Input: part model. Units: mm. Frame: model coordinates. A direction names the side the tool comes from. Coordinates: 2 decimals unless noted, no trailing zeros. Order: outer loops, then holes, each group sorted by start corner. A loop starts at its lowest first (then second) coordinate and runs counter-clockwise, first axis right, second up. Notation, with made-up numbers: M 34.5,34 L 67.5,34 A22 cw 67.5,71 Z; hole C -38,15.5 d4. An arc over 180 degrees is marked long. One line per item, written item: value.
```python
from build123d import *

# Parameters (mm, degrees)
SKETCH_1_R               = 130
SKETCH_1_R_2             = 30
SKETCH_1_R_3             = 2.1
SKETCH_1_R_4             = 1.6
EXTRUDE_1_DEPTH          = 5
SKETCH_2_R               = 1.4
CUT_EXTRUDE_1_DEPTH      = 1
CUT_EXTRUDE_1_DEPTH_BACK = 6
CUT_EXTRUDE_2_REACH      = 7
SKETCH_8_R               = 1.6
CUT_EXTRUDE_3_DEPTH      = 314.847763109


with BuildPart() as part:
    # 草图1 → 凸台-拉伸1 (new body)
    with BuildSketch(Plane.XY):
        Circle(SKETCH_1_R)
        Circle(SKETCH_1_R_2, mode=Mode.SUBTRACT)
        with Locations((0, 120)):
            Circle(SKETCH_1_R_3, mode=Mode.SUBTRACT)
        with Locations((120, 0)):
            Circle(SKETCH_1_R_3, mode=Mode.SUBTRACT)
        with Locations((0, -120)):
            Circle(SKETCH_1_R_3, mode=Mode.SUBTRACT)
        with Locations((-120, 0)):
            Circle(SKETCH_1_R_3, mode=Mode.SUBTRACT)
        with Locations((0, 40)):
            Circle(SKETCH_1_R_4, mode=Mode.SUBTRACT)
        with Locations((40, 0)):
            Circle(SKETCH_1_R_4, mode=Mode.SUBTRACT)
        with Locations((0, -40)):
            Circle(SKETCH_1_R_4, mode=Mode.SUBTRACT)
        with Locations((-40, 0)):
            Circle(SKETCH_1_R_4, mode=Mode.SUBTRACT)
    extrude(amount=EXTRUDE_1_DEPTH)

    # 草图2 → 切除-拉伸1 (cut, two sides)
    with BuildSketch(Plane.XY.offset(5)) as cut_extrude_1_sk:
        with Locations((0, 95)):
            Circle(SKETCH_2_R)
        with Locations((15, 80)):
            Circle(SKETCH_2_R)
        with Locations((0, 65)):
            Circle(SKETCH_2_R)
        with Locations((-15, 80)):
            Circle(SKETCH_2_R)
        with Locations((95, 0)):
            Circle(SKETCH_2_R)
        with Locations((80, -15)):
            Circle(SKETCH_2_R)
        with Locations((65, 0)):
            Circle(SKETCH_2_R)
        with Locations((80, 15)):
            Circle(SKETCH_2_R)
        with Locations((0, -95)):
            Circle(SKETCH_2_R)
        with Locations((-15, -80)):
            Circle(SKETCH_2_R)
        with Locations((0, -65)):
            Circle(SKETCH_2_R)
        with Locations((15, -80)):
            Circle(SKETCH_2_R)
        with Locations((-95, 0)):
            Circle(SKETCH_2_R)
        with Locations((-80, 15)):
            Circle(SKETCH_2_R)
        with Locations((-65, 0)):
            Circle(SKETCH_2_R)
        with Locations((-80, -15)):
            Circle(SKETCH_2_R)
    extrude(amount=CUT_EXTRUDE_1_DEPTH, mode=Mode.SUBTRACT)
    extrude(cut_extrude_1_sk.sketch, amount=-CUT_EXTRUDE_1_DEPTH_BACK, mode=Mode.SUBTRACT)

    # 草图8 → 切除-拉伸2 (cut, up to next)
    with BuildSketch(Plane(origin=(0, 0, 0), x_dir=(-1, 0, 0), z_dir=(0, 0, -1)), mode=Mode.PRIVATE) as cut_extrude_2_sk1:
        with Locations((-75.840860977, 86.447462694)):
            Circle(SKETCH_8_R)
    cut_extrude_2_tool1 = extrude(cut_extrude_2_sk1.sketch, amount=-CUT_EXTRUDE_2_REACH, mode=Mode.PRIVATE) & part.part
    add(cut_extrude_2_tool1.solids().sort_by_distance((75.840861, 86.447463, 0))[0], mode=Mode.SUBTRACT)
    # 草图8 → 切除-拉伸2 (cut, up to next)
    with BuildSketch(Plane(origin=(0, 0, 0), x_dir=(-1, 0, 0), z_dir=(0, 0, -1)), mode=Mode.PRIVATE) as cut_extrude_2_sk2:
        with Locations((-86.447462694, 75.840860977)):
            Circle(SKETCH_8_R)
    cut_extrude_2_tool2 = extrude(cut_extrude_2_sk2.sketch, amount=-CUT_EXTRUDE_2_REACH, mode=Mode.PRIVATE) & part.part
    add(cut_extrude_2_tool2.solids().sort_by_distance((86.447463, 75.840861, 0))[0], mode=Mode.SUBTRACT)
    # 草图8 → 切除-拉伸2 (cut, up to next)
    with BuildSketch(Plane(origin=(0, 0, 0), x_dir=(-1, 0, 0), z_dir=(0, 0, -1)), mode=Mode.PRIVATE) as cut_extrude_2_sk3:
        with Locations((-65.948574762, 75.171706691)):
            Circle(SKETCH_8_R)
    cut_extrude_2_tool3 = extrude(cut_extrude_2_sk3.sketch, amount=-CUT_EXTRUDE_2_REACH, mode=Mode.PRIVATE) & part.part
    add(cut_extrude_2_tool3.solids().sort_by_distance((65.948575, 75.171707, 0))[0], mode=Mode.SUBTRACT)
    # 草图8 → 切除-拉伸2 (cut, up to next)
    with BuildSketch(Plane(origin=(0, 0, 0), x_dir=(-1, 0, 0), z_dir=(0, 0, -1)), mode=Mode.PRIVATE) as cut_extrude_2_sk4:
        with Locations((-75.171706691, 65.948574762)):
            Circle(SKETCH_8_R)
    cut_extrude_2_tool4 = extrude(cut_extrude_2_sk4.sketch, amount=-CUT_EXTRUDE_2_REACH, mode=Mode.PRIVATE) & part.part
    add(cut_extrude_2_tool4.solids().sort_by_distance((75.171707, 65.948575, 0))[0], mode=Mode.SUBTRACT)
    # 草图8 → 切除-拉伸2 (cut, up to next)
    with BuildSketch(Plane(origin=(0, 0, 0), x_dir=(-1, 0, 0), z_dir=(0, 0, -1)), mode=Mode.PRIVATE) as cut_extrude_2_sk5:
        with Locations((65.948574762, -75.171706691)):
            Circle(SKETCH_8_R)
    cut_extrude_2_tool5 = extrude(cut_extrude_2_sk5.sketch, amount=-CUT_EXTRUDE_2_REACH, mode=Mode.PRIVATE) & part.part
    add(cut_extrude_2_tool5.solids().sort_by_distance((-65.948575, -75.171707, 0))[0], mode=Mode.SUBTRACT)
    # 草图8 → 切除-拉伸2 (cut, up to next)
    with BuildSketch(Plane(origin=(0, 0, 0), x_dir=(-1, 0, 0), z_dir=(0, 0, -1)), mode=Mode.PRIVATE) as cut_extrude_2_sk6:
        with Locations((75.171706691, -65.948574762)):
            Circle(SKETCH_8_R)
    cut_extrude_2_tool6 = extrude(cut_extrude_2_sk6.sketch, amount=-CUT_EXTRUDE_2_REACH, mode=Mode.PRIVATE) & part.part
    add(cut_extrude_2_tool6.solids().sort_by_distance((-75.171707, -65.948575, 0))[0], mode=Mode.SUBTRACT)
    # 草图8 → 切除-拉伸2 (cut, up to next)
    with BuildSketch(Plane(origin=(0, 0, 0), x_dir=(-1, 0, 0), z_dir=(0, 0, -1)), mode=Mode.PRIVATE) as cut_extrude_2_sk7:
        with Locations((75.840860977, -86.447462694)):
            Circle(SKETCH_8_R)
    cut_extrude_2_tool7 = extrude(cut_extrude_2_sk7.sketch, amount=-CUT_EXTRUDE_2_REACH, mode=Mode.PRIVATE) & part.part
    add(cut_extrude_2_tool7.solids().sort_by_distance((-75.840861, -86.447463, 0))[0], mode=Mode.SUBTRACT)
    # 草图8 → 切除-拉伸2 (cut, up to next)
    with BuildSketch(Plane(origin=(0, 0, 0), x_dir=(-1, 0, 0), z_dir=(0, 0, -1)), mode=Mode.PRIVATE) as cut_extrude_2_sk8:
        with Locations((86.447462694, -75.840860977)):
            Circle(SKETCH_8_R)
    cut_extrude_2_tool8 = extrude(cut_extrude_2_sk8.sketch, amount=-CUT_EXTRUDE_2_REACH, mode=Mode.PRIVATE) & part.part
    add(cut_extrude_2_tool8.solids().sort_by_distance((-86.447463, -75.840861, 0))[0], mode=Mode.SUBTRACT)

    # 草图5 → 切除-拉伸3 (cut, through all)
    with BuildSketch(Plane(origin=(91.923881554, 91.923881554, 0), x_dir=(0, 0, -1), z_dir=(0.707106781, 0.707106781, 0))):
        Polygon((0, -10), (-2.5, -10), (-2.5, 10), (-5, 10), (-5, 130), (0, 130), align=None)
    extrude(amount=-CUT_EXTRUDE_3_DEPTH, mode=Mode.SUBTRACT)


solid = part.part
```
(1) Cut plane C-C on y = -46. Output: boundary loops of the cut face in (x, z).
Data:
outline: M -60.14,2.5 L -31.86,2.5 L -31.86,0 L 121.59,0 L 121.59,5 L -60.14,5 Z
(2) Draft query along Y for faces 1 (the cylindrical face through (20.64, -21.77, 3.02)), 2 (the flat face through (57, 56, 2.5)), 3 (the flat face through (63.4, 49.26, 1.23)). Return one class per face: released by +Y, released by -Y, zero draft, split by the parting line, or undercut.
Data:
face 1: undercut
face 2: zero draft
face 3: released by +Y
(3) Access query for faces 4 (the flat face through (39, -39, 5)), 5 (the flat face through (-55, -56, 2.5)). Directions: +Z, -Z, +X, -X, +Y, -Y. A direction counts if a zero-diameter tool reaches every point of the face in a straight line with its end or side. Return the directions, or none.
Data:
face 4: +Z, +X, -X, +Y, -Y
face 5: -Z, -X, +Y
(4) Ray query, line 1 (Y direction, x = 0, z = 2.15); line 2 (X direction, y = -79.5, z = 4.2); line 3 (Y direction, x = 40, z = 1.1). Return the intervals inside material, ascending. Write a range as from..to.
Data:
line 1: y = -130..-122.1, -117.9..-96.4, -93.6..-66.4, -63.6..-41.6, -38.4..-30
line 2: x = -93.64..-16.31, -13.69..13.69, 16.31..102.86
line 3: y = -123.69..-1.6, 1.6..25.86
(5) First-contact query: pin 1 (3.5 mm diameter, centred on x = 80, y = -15, fed in from -Z); pin 2 (4 mm diameter, centred on x = 75.84, y = 86.45, fed in from -Z); pin 3 (1.5 mm diameter, centred on y = 18.5, z = 3.5, fed in from +X). Flat tips, straight axial feed; report the tip coordinate or a pass-through.
Data:
pin 1: stops at z = 0
pin 2: stops at z = 2.5
pin 3: stops at x = 128.78
(6) Cut plane B-B on x = -51. Output: boundary loops of the cut face in (y, z), plus the area to 3 significant figures.
Data:
outline: M -119.58,0 L -65.14,0 L -65.14,2.5 L -36.86,2.5 L -36.86,5 L -119.58,5 Z
area: 343 mm2
(7) Cut plane D-D on x = 109.5. Output: boundary loops of the cut face in (y, z), plus the area to 3 significant figures.
Data:
outline: M -70.07,0 L 70.07,0 L 70.07,5 L -70.07,5 Z
area: 701 mm2
(8) Cut plane A-A on z = 1.75. Give the number of separate pieces and of enclosed holes in the cut face, plus the area to 3 significant figures.
Data:
separate pieces: 1
enclosed holes: 12
area: 23,000 mm2
